```python
from build123d import *

# Parameters (mm, degrees)
F0_W          = 44.45
F0_H          = 187.96
F1_DEPTH      = 46.355
F2_R          = 5.08
F3_W          = 34.29
F3_H          = 38.1
F4_DEPTH      = 5.08
F5_R          = 12.7
F6_DEPTH      = 2.54
F7_W          = 31.75
F7_H          = 7.62
F8_DEPTH      = 7.62
F9_W          = 31.75
F9_H          = 7.62
F10_DEPTH     = 7.62
F11_W         = 25.4
F11_H         = 7.62
F12_DEPTH     = 7.62
F13_W         = 25.4
F13_H         = 7.62
F14_DEPTH     = 7.62
F15_SIZE      = 3.81
F16_T         = 5.08
F16_T3_DEPTH  = 44.45
F16_T5_DEPTH  = 48.26
F16_T7_DEPTH  = 35.56
F16_T9_DEPTH  = 17.78
F16_T11_DEPTH = 41.91
F17_W         = 34.29
F17_H         = 69.85
F18_DEPTH     = 25.4
F19_R         = 3.302
F20_DEPTH     = 53.976


# Not quite as in the source:
# - a shell that OpenCascade refuses in one call is made with other operations: the cavity is built on its own and cut out


with BuildPart() as f1:
    # F0 (on Top) → F1 (new body)
    with BuildSketch(Plane.XY):
        Rectangle(F0_W, F0_H)
    extrude(amount=F1_DEPTH)

    # F2
    f2_edges = [f1.edges().sort_by_distance(p)[0] for p in [
        (22.225, 0, 46.355),
        (-22.225, 0, 46.355),
    ]]
    fillet(f2_edges, radius=F2_R)

    # F3 (on face) → F4 (join)
    with BuildSketch(Plane.XY.offset(46.355)):
        with Locations((0, 50.8)):
            Rectangle(F3_W, F3_H)
    extrude(amount=F4_DEPTH)

    # F5 (on face) → F6 (join)
    with BuildSketch(Plane.XY.offset(51.435)):
        with Locations((0, 50.8)):
            Circle(F5_R)
    extrude(amount=F6_DEPTH)

    # F7 (on face) → F8 (join)
    with BuildSketch(Plane.YZ.offset(22.225)):
        with Locations((15.875, 3.81)):
            Rectangle(F7_W, F7_H)
    extrude(amount=F8_DEPTH)

    # F9 (on face) → F10 (join)
    with BuildSketch(Plane(origin=(-22.225, 0, 0), x_dir=(0, -1, 0), z_dir=(-1, 0, 0))):
        with Locations((-15.875, 3.81)):
            Rectangle(F9_W, F9_H)
    extrude(amount=F10_DEPTH)

    # F11 (on face) → F12 (join)
    with BuildSketch(Plane(origin=(-22.225, 0, 0), x_dir=(0, -1, 0), z_dir=(-1, 0, 0))):
        with Locations((-81.28, 3.81)):
            Rectangle(F11_W, F11_H)
    extrude(amount=F12_DEPTH)

    # F13 (on face) → F14 (join)
    with BuildSketch(Plane.YZ.offset(22.225)):
        with Locations((81.28, 3.81)):
            Rectangle(F13_W, F13_H)
    extrude(amount=F14_DEPTH)

    # F15
    f15_edges = [f1.edges().sort_by_distance(p)[0] for p in [
        (-17.145, 50.8, 51.435),
        (17.145, 50.8, 51.435),
    ]]
    chamfer(f15_edges, length=F15_SIZE)

    # F16: shell of thickness 5.08, made by hand


with BuildPart() as f16_core1:
    # F16_t2: copy of F1
    add(f1.part)

    # the walls: a layer under each face that stays
    f16_faces = [f16_core1.faces().sort_by_distance(p)[0] for p in [
        (0, 31.75, 48.895),
        (-17.145, 50.8, 46.99),
        (-15.24, 50.8, 49.53),
        (0, -31.115, 46.355),
        (-8.89, 38.1, 51.435),
        (17.145, 50.8, 46.99),
        (15.24, 50.8, 49.53),
        (0, 69.85, 48.895),
        (0, -93.98, 23.1775),
        (-12.7, 50.8, 52.705),
        (0, 81.915, 46.355),
        (0, 93.98, 23.1775),
        (-22.225, 0, 20.6375),
        (22.225, 0, 20.6375),
        (0, 50.8, 53.975),
        (-26.035, 81.28, 7.62),
        (-29.845, 81.28, 3.81),
        (29.845, 81.28, 3.81),
        (26.035, 81.28, 7.62),
        (-26.035, 68.58, 3.81),
        (-26.035, 31.75, 3.81),
        (-26.035, 15.875, 7.62),
        (-26.035, 0, 3.81),
        (26.035, 0, 3.81),
        (26.035, 15.875, 7.62),
        (26.035, 31.75, 3.81),
        (26.035, 68.58, 3.81),
        (-29.845, 15.875, 3.81),
        (29.845, 15.875, 3.81),
    ]]
    thicken(f16_faces, amount=-F16_T, mode=Mode.SUBTRACT)

    # F16_s4 → F16_t3 (cut)
    with BuildSketch(Plane.YZ.offset(-22.225)):
        Polygon((31.6992, 46.4058), (36.83, 46.355), (36.83, 41.275), (31.75, 41.275), align=None)
        Polygon((69.9008, 46.4058), (64.77, 46.355), (64.77, 41.275), (69.85, 41.275), align=None)
    extrude(amount=F16_T3_DEPTH, mode=Mode.SUBTRACT)

    # F16_s6 → F16_t5 (cut)
    with BuildSketch(Plane.XZ.offset(-74.93)):
        Polygon((-17.1958, 46.4058), (-12.065, 46.355), (-12.065, 41.275), (-17.145, 41.275), align=None)
        Polygon((17.1958, 46.4058), (12.065, 46.355), (12.065, 41.275), (17.145, 41.275), align=None)
    extrude(amount=F16_T5_DEPTH, mode=Mode.SUBTRACT)

    # F16_s8 → F16_t7 (cut)
    with BuildSketch(Plane.XZ.offset(-99.06)):
        Polygon((-22.2758, 7.6708), (-17.145, 7.62), (-17.145, 2.54), (-22.225, 2.54), align=None)
        Polygon((22.2758, 7.6708), (17.145, 7.62), (17.145, 2.54), (22.225, 2.54), align=None)
    extrude(amount=F16_T7_DEPTH, mode=Mode.SUBTRACT)

    # F16_s10 → F16_t9 (cut)
    with BuildSketch(Plane.XY.offset(-5.08)):
        Polygon((-22.2758, 68.5292), (-17.145, 68.58), (-17.145, 73.66), (-22.225, 73.66), align=None)
        Polygon((-22.2758, 31.8008), (-17.145, 31.75), (-17.145, 26.67), (-22.225, 26.67), align=None)
        Polygon((-22.2758, -0.0508), (-17.145, 0), (-17.145, 5.08), (-22.225, 5.08), align=None)
        Polygon((22.2758, -0.0508), (17.145, 0), (17.145, 5.08), (22.225, 5.08), align=None)
        Polygon((22.2758, 31.8008), (17.145, 31.75), (17.145, 26.67), (22.225, 26.67), align=None)
        Polygon((22.2758, 68.5292), (17.145, 68.58), (17.145, 73.66), (22.225, 73.66), align=None)
    extrude(amount=F16_T9_DEPTH, mode=Mode.SUBTRACT)

    # F16_s12 → F16_t11 (cut)
    with BuildSketch(Plane.XZ.offset(-36.83)):
        Polygon((-22.2758, 7.6708), (-17.145, 7.62), (-17.145, 2.54), (-22.225, 2.54), align=None)
        Polygon((22.2758, 7.6708), (17.145, 7.62), (17.145, 2.54), (22.225, 2.54), align=None)
    extrude(amount=F16_T11_DEPTH, mode=Mode.SUBTRACT)

    # F16_s13 → F16_t14 (revolve, cut)
    with BuildSketch(Plane.XZ.offset(-50.8)):
        Polygon((12.7508, 51.4858), (12.7, 46.355), (7.62, 46.355), (7.62, 51.435), align=None)
    revolve(axis=Axis((0, 50.8, 51.435), (0, 0, 1)), mode=Mode.SUBTRACT)


with BuildPart() as f1_1:
    add(f1.part)

    # what is left inside the walls is the cavity
    f16_cavity = [f16_core1.part.solids().sort_by_distance(p)[0] for p in [
        (17.0942, 0, 27.516667),
    ]]
    add(f16_cavity, mode=Mode.SUBTRACT)

    # F17 (on face) → F18 (cut)
    with BuildSketch(Plane.XY.offset(46.355)):
        with Locations((0, -6.35)):
            Rectangle(F17_W, F17_H)
    extrude(amount=-F18_DEPTH, mode=Mode.SUBTRACT)

    # F19 (on face) → F20 (cut, through all)
    with BuildSketch(Plane.XY.offset(53.975)):
        with Locations((0, 50.8)):
            Circle(F19_R)
    extrude(amount=-F20_DEPTH, mode=Mode.SUBTRACT)


solid = f1_1.part
```
Verification items for the finished model (mm, model axes). A direction names the side the tool comes from. Coordinates: 2 decimals unless noted, no trailing zeros. Write each loop counter-clockwise with the first axis right and the second up, starting at its lowest first coordinate (ties: lowest second). Pieces come first, ordered by that corner, then holes. Notation, with made-up numbers: (-12.75, 4) - (18.25, 4) arc R30 cw to (18.25, 38) - close; hole circle Ø8 at (2, 5.5). An arc over 180 degrees is marked (long way). One line per question, with ' | ' between items. Start each with the question number.
1. Material ranges on line 1 along X through (y, z) = (48, 32) (3 decimals); line 2 along Y through (x, z) = (-2, 33.5); line 3 along Y through (x, z) = (2.5, 42) (3 decimals), recorded low to high.
2. Section check B-B (z = 27.5). Enter the section's corners in (x, y) (3 decimals), plus the area to 3 significant figures.
3. Draft check along Y on faces 1 (the flat face through (-21, 81, 2.54)), 2 (the flat face through (0, 30, 46.355)), 3 (the flat face through (26, 0, 4)). Enter one of: released by +Y, released by -Y, zero draft, split by the parting line, or undercut.
4. Section check A-A (x = 0). Count the separate pieces of the cut face and the enclosed holes in it, plus the area to 3 significant figures.
5. Section check C-C (y = -25.5). Enter the section's corners in (x, z) (3 decimals), plus the area to 3 significant figures.
6. Access from +Z, -Z, +X, -X, +Y, -Y to the whole of each face (thin tool, end or side, straight path). Record for faces 4 (the flat face through (0, 65, 41.275)), 5 (the flat face through (0, -67, 46.355)), 6 (the flat face through (26, 68.58, 4)), 7 (the flat face through (-26, 68.58, 4)).
7. Gauge pin test, flat ends, axial feed: P1, Ø3, axis at x = 9, y = 34.5, coming from the +Z side (3 decimals); P2, Ø8.5, axis at x = 25.5, y = 80, coming from the +Z side; P3, Ø2.5, axis at x = 24, y = 15, coming from the +Z side; P4, Ø1, axis at x = 16.5, y = -27, coming from the -Z side. Record the tip position at first contact, or that the pin passes through.
Computed values:
1) line 1: -22.225 to -17.145, 17.145 to 22.225 | line 2: -93.98 to -88.9, 88.9 to 93.98 | line 3: -93.98 to -41.275, 28.575 to 36.83, 64.77 to 93.98
2) outline: (-22.225, -93.98) - (22.225, -93.98) - (22.225, 93.98) - (-22.225, 93.98) - close; hole (-17.145, -88.9) - (17.145, -88.9) - (17.145, 88.9) - (-17.145, 88.9) - close | area: 2,260 mm²
3) face 1: undercut | face 2: zero draft | face 3: released by -Y
4) separate pieces: 3 | enclosed holes: 0 | area: 1,060 mm²
5) outline: (-22.225, 0) - (-17.145, 0) - (-17.145, 46.355) arc R5.08 ccw to (-22.225, 41.275) - close; (17.145, 0) - (22.225, 0) - (22.225, 41.275) arc R5.08 ccw to (17.145, 46.355) - close | area: 460 mm²
6) face 4: -Z | face 5: +Z, +X, -X, -Y | face 6: +Z, -Z, +X | face 7: +Z, -Z, -X
7) P1: z = 51.435 | P2: z = 44.27 | P3: z = 7.62 | P4: through
